Geometry check sheet. Reference: the model listing, model coordinates, mm. Face numbers are marked on the shaded views. Coordinates: 2 decimals unless noted, no trailing zeros. Loops run counter-clockwise (first coordinate to the right, second up) from the corner with the lowest first, then second, coordinate; pieces in that order, holes last. Notation, with made-up numbers: (51.5, 29.25) - (93.5, 29.25) arc R26 cw to (93.5, 57.25) - close; hole circle Ø11 at (52.5, -13). An arc over 180 degrees is marked (long way). Write each question's results on one line, items separated by ' | '. Start each with the question number.
(1) Go/stop test with flat-tipped pins: pin 1 Ø2 at (y, z) = (-7.5, 8.5) entering from -X; pin 2 Ø1.5 at (y, z) = (-1, 6) entering from +X; pin 3 Ø1 at (x, z) = (-3.5, 4.5) entering from +Y. Record where each tip stops, or that it passes through.
(2) Sectioned sample at A-A (x = 0). Enter the section's corners in (y, z), plus the area to 3 significant figures.
(3) Material ranges on probe 1 along X at (y, z) = (-3.25, 6); probe 2 along Y at (x, z) = (0, 0.4); probe 3 along X at (y, z) = (0, 0.6), recorded low to high.
(4) Sectioned sample at C-C (z = 7.25). Enter the section's corners in (x, y).
(5) Mould release check, pull along Y, two halves, no side actions. Record for the marked faces 1, 2 and 3: pulls with the +Y half, pulls with the -Y half, needs draft (parallel to the pull), parting line crosses it, or undercut.
(6) Sectioned sample at D-D (z = 9). Enter the section's corners in (x, y).
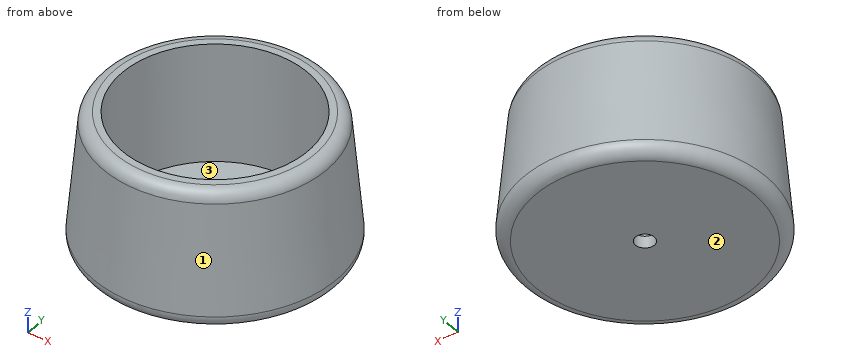
from build123d import *


with BuildPart() as f1:
    # F0 (on Front) → F1 (revolve)
    with BuildSketch(Plane.XZ):
        with BuildLine():
            Line((-9.204967, 0), (-0.8, 0))
            Line((-0.8, 0), (-0.8, 1))
            Line((-0.8, 1), (-7.8, 1))
            Line((-7.8, 1), (-7.8, 11))
            Line((-7.8, 11), (-8.386785, 11))
            ThreePointArc((-8.386785, 11), (-9.061124, 10.738423), (-9.382679, 10.090536))
            Line((-9.382679, 10.090536), (-10.20086, 1.090536))
            ThreePointArc((-10.20086, 1.090536), (-9.94339, 0.325662), (-9.204967, 0))
        make_face()
    revolve(axis=Axis((0, 0, 1.31524), (0, 0, 1)))


solid = f1.part
Outcome:
1) pin 1: stops at x = -6.97 | pin 2: stops at x = 9.79 | pin 3: stops at y = 9.43
2) outline: (-10.2, 1.09) arc R1 ccw to (-9.2, 0) - (-0.8, 0) - (-0.8, 1) - (-7.8, 1) - (-7.8, 11) - (-8.39, 11) arc R1 ccw to (-9.38, 10.09) - close; (0.8, 0) - (9.2, 0) arc R1 ccw to (10.2, 1.09) - (9.38, 10.09) arc R1 ccw to (8.39, 11) - (7.8, 11) - (7.8, 1) - (0.8, 1) - close | area: 57.1 mm2
3) probe 1: x = -9.2 to -7.09, 7.09 to 9.2 | probe 2: y = -10 to -0.8, 0.8 to 10 | probe 3: x = -10.12 to -0.8, 0.8 to 10.12
4) outline: circle Ø19.28 at (0, 0); hole circle Ø15.6 at (0, 0)
5) face 1: parting line crosses it | face 2: needs draft | face 3: undercut
6) outline: circle Ø18.96 at (0, 0); hole circle Ø15.6 at (0, 0)
